Work out the finished part from the listing and answer in its coordinate system (mm). Round coordinates to 2 decimals unless told otherwise and drop trailing zeros. Loops run counter-clockwise (first coordinate to the right, second up) from the corner with the lowest first, then second, coordinate; pieces in that order, holes last.
Autodesk Inventor part; units mm, degrees
ref_plane "YZ Plane" through (0, 0, 0) normal (1, 0, 0) x (0, 1, 0)
ref_plane "XZ Plane" through (0, 0, 0) normal (0, 1, 0) x (-1, 0, 0)
ref_plane "XY Plane" through (0, 0, 0) normal (0, 0, 1) x (1, 0, 0)
sketch "Sketch1" plane through (0, 0, 0) normal (0, 1, 0) x (-1, 0, 0)
  line L0 (-25, 25) -> (25, 25)
  line L1 (25, 25) -> (25, -25)
  line L2 (25, -25) -> (-25, -25)
  line L3 (-25, -25) -> (-25, 25)
  line L4 (-25, 25) -> (25, -25) construction
  line L5 (25, 25) -> (-25, -25) construction
  point P0 (0, 0)
  dimension "d0" = 50
  dimension "d1" = 50
extrude "Extrusion1" add sketch "Sketch1" along normal blind 1.6
sketch "Sketch2" plane through (0, 1.6, 0) normal (0, 1, 0) x (1, 0, 0)
  circle A0 centre (-23, -19) radius 1
  line L0 (-25, 25) -> (-25, -25)
  line L1 (-25, -25) -> (25, -25)
  circle A1 centre (19, -23) radius 1
  circle A2 centre (23, 19) radius 1
  circle A3 centre (-19, 23) radius 1
  line L2 (25, -25) -> (25, 25)
  line L3 (25, 25) -> (-25, 25)
  point P0 (0, 0)
  dimension "d4" = 2
  dimension "d5" = 2
  dimension "d6" = 6
  dimension "d7" = 2
  dimension "d8" = 2
  dimension "d9" = 2
  dimension "d10" = 2
  dimension "d11" = 6
  dimension "d12" = 6
  dimension "d13" = 2
  dimension "d14" = 2
  dimension "d15" = 6
extrude "Extrusion2" cut sketch "Sketch2" against normal blind 2 contours A0 | A1 | A2 | A3
sketch "Sketch3" plane through (0, 1.6, 0) normal (0, 1, 0) x (1, 0, 0)
  circle A0 centre (0, 1.3) radius 0.5
  circle A1 centre (0, -1.3) radius 0.5
  point P0 (0, 0)
  dimension "d18" = 1
  dimension "d19" = 1
  dimension "d20" = 1.3
  dimension "d21" = 1.3
extrude "Extrusion3" cut sketch "Sketch3" against normal blind 2
equation "\"d16\" = d14"
properties part number "Solar Panel PCB" material "ABS Plastic"
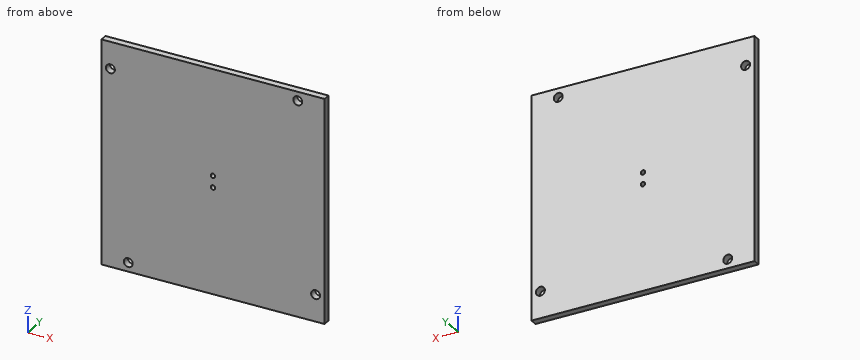
1. Find section A-A (x = 19). Write down the section's boundary in (y, z).
Answer key:
outline: (0, -25) - (1.6, -25) - (1.6, 22) - (0, 22) - close; (0, 24) - (1.6, 24) - (1.6, 25) - (0, 25) - close
2. Consider probe 1 along X at (y, z) = (1.25, 19); probe 2 along Z at (x, y) = (19, 0.5); probe 3 along X at (y, z) = (1.15, 23). Determine where each line is inside the solid, lowest interval first.
Answer key:
probe 1: x = -25 to -24, -22 to 25
probe 2: z = -25 to 22, 24 to 25
probe 3: x = -25 to 18, 20 to 25
3. Find section B-B (z = -23). Write down the section's boundary in (x, y).
Answer key:
outline: (-25, 0) - (-20, 0) - (-20, 1.6) - (-25, 1.6) - close; (-18, 0) - (25, 0) - (25, 1.6) - (-18, 1.6) - close
